```python
from build123d import *
from OCP.BRepFilletAPI import BRepFilletAPI_MakeChamfer

# Parameters (mm, degrees)
SKETCH1_W           = 60.96
SKETCH1_H           = 16.51
SKETCH1_W_2         = 50.8
SKETCH1_H_2         = 6.35
BOSS_EXTRUDE1_DEPTH = 19.05
BOSS_EXTRUDE2_DEPTH = 60.96
SKETCH7_W           = 50.8
SKETCH7_H           = 6.35
CUT_EXTRUDE1_DEPTH  = 19.05
SKETCH8_R           = 1.524
CUT_EXTRUDE2_DEPTH  = 61.718810561
SKETCH9_R           = 1.593897105
CUT_EXTRUDE3_DEPTH  = 69.202157429
CHAMFER1_SIZE       = 2.1082
CHAMFER1_SIZE2      = 1.832630301
SKETCH10_W          = 52.07
SKETCH10_H          = 7.62
CUT_EXTRUDE4_DEPTH  = 19.05
SKETCH11_W          = 52.07
SKETCH11_H          = 7.62
CUT_EXTRUDE5_DEPTH  = 19.05
CHAMFER2_SIZE       = 1.27


with BuildPart() as part:
    # Sketch1 → Boss-Extrude1 (new body)
    with BuildSketch(Plane(origin=(0, 0, 0), x_dir=(1, 0, 0), z_dir=(0, 1, 0))):
        Rectangle(SKETCH1_W, SKETCH1_H)
        Rectangle(SKETCH1_W_2, SKETCH1_H_2, mode=Mode.SUBTRACT)
    extrude(amount=BOSS_EXTRUDE1_DEPTH)

    # Sketch5 → Boss-Extrude2 (add)
    with BuildSketch(Plane(origin=(30.48, 0, 0), x_dir=(0, 0, -1), z_dir=(1, 0, 0))):
        with BuildLine():
            Line((8.255, 19.05), (-8.255, 19.05))
            Line((-8.255, 19.05), (-39.884181664, 16.282805168))
            Line((-39.884181664, 16.282805168), (-41.323122977, 32.729979633))
            Line((-41.323122977, 32.729979633), (-28.671450311, 33.836857566))
            Line((-28.671450311, 33.836857566), (-9.693941313, 35.497174465))
            ThreePointArc((-9.693941313, 35.497174465), (2.898994328, 31.222448831), (8.255, 19.05))
        make_face()
    extrude(amount=-BOSS_EXTRUDE2_DEPTH)

    # Sketch7 → Cut-Extrude1 (cut)
    with BuildSketch(Plane(origin=(0, -3.339221533, 38.167476773), x_dir=(1, 0, 0), z_dir=(0, -0.08715574274765728, 0.9961946980917457))):
        with Locations((0, 28.449053402)):
            Rectangle(SKETCH7_W, SKETCH7_H)
    extrude(amount=-CUT_EXTRUDE1_DEPTH, mode=Mode.SUBTRACT)

    # Sketch8 → Cut-Extrude2 (cut, through all)
    with BuildSketch(Plane(origin=(0, 36.069201166, 3.155646204), x_dir=(1, 0, 0), z_dir=(0, 0.9961946980917459, 0.08715574274765486))):
        with Locations(Location((0, -28.153270333, 0), (0, 0, 270))):
            Circle(SKETCH8_R)
    extrude(amount=-CUT_EXTRUDE2_DEPTH, mode=Mode.SUBTRACT)

    # Sketch9 → Cut-Extrude3 (cut, through all)
    with BuildSketch(Plane(origin=(0, 0, -8.255), x_dir=(-1, 0, 0), z_dir=(0, 0, -1))):
        with Locations((0, 10.16)):
            Circle(SKETCH9_R)
    extrude(amount=-CUT_EXTRUDE3_DEPTH, mode=Mode.SUBTRACT)

    # Chamfer1: one chamfer whose edges measure the first distance from different faces: ONE call of the kernel's chamfer builder (chamfer() names one face for all edges)
    chamfer1_edges_1 = [part.edges().sort_by_distance(p)[0] for p in [
        (0, 33.748307332, 29.683584125),
    ]]
    chamfer1_side_1 = [part.faces().sort_by_distance(p)[0] for p in [
        (0, 34.115461929, 25.486987868),
    ]]
    chamfer1_edges_2 = [part.edges().sort_by_distance(p)[0] for p in [
        (1.593897105, 10.16, -8.255),
    ]]
    chamfer1_side_2 = [part.faces().sort_by_distance(p)[0] for p in [
        (-29.841327619, 9.525, -8.255),
    ]]
    chamfer1 = BRepFilletAPI_MakeChamfer(part.part.solid().wrapped)
    for e in chamfer1_edges_1:
        chamfer1.Add(CHAMFER1_SIZE, CHAMFER1_SIZE2, e.wrapped, chamfer1_side_1[0].wrapped)  # the first distance lies on this face
    for e in chamfer1_edges_2:
        chamfer1.Add(CHAMFER1_SIZE, CHAMFER1_SIZE2, e.wrapped, chamfer1_side_2[0].wrapped)  # the first distance lies on this face
    add(Compound.cast(chamfer1.Shape()), mode=Mode.REPLACE)

    # Sketch10 → Cut-Extrude4 (cut)
    with BuildSketch(Plane(origin=(0, -3.339221533, 38.167476773), x_dir=(1, 0, 0), z_dir=(0, -0.08715574274765728, 0.9961946980917457))):
        with Locations((0, 28.449053402)):
            Rectangle(SKETCH10_W, SKETCH10_H)
    extrude(amount=-CUT_EXTRUDE4_DEPTH, mode=Mode.SUBTRACT)

    # Sketch11 → Cut-Extrude5 (cut)
    with BuildSketch(Plane.XZ):
        Rectangle(SKETCH11_W, SKETCH11_H)
    extrude(amount=-CUT_EXTRUDE5_DEPTH, mode=Mode.SUBTRACT)

    # Chamfer2
    chamfer2_edges = [part.edges().sort_by_distance(p)[0] for p in [
        (30.48, 31.222448831, -2.898994328),
        (30.48, 34.113577049, 25.508532145),
        (-30.48, 31.222448831, -2.898994328),
        (-30.48, 34.113577049, 25.508532145),
        (-30.48, 9.525, -8.255),
        (30.48, 9.525, -8.255),
    ]]
    chamfer(chamfer2_edges, length=CHAMFER2_SIZE)


solid = part.part
```
Build history of the part. All positions in model axes, mm. A direction names the side the tool comes from. Give positions to 0.01 mm unless a question says otherwise; leave off trailing zeros. Order: outer loops, then holes, each group sorted by start corner. A loop starts at its lowest first (then second) coordinate and runs counter-clockwise, first axis right, second up. Notation, with made-up numbers: M 36,16.5 L 69,16.5 A21 cw 69,29.5 Z; hole C -6.75,43 d3. An arc over 180 degrees is marked long. Return JSON: item names as keys, results as strings.
Q1. Two-plate mould, pull along Z, no slides. Class faces 1 (the face through (-30.48, 21, 12)), 2 (the face through (-0.36, 21.84, 33.07)), 3 (the face through (0.427, 17.686, 23.848)): pulls with the +Z half, pulls with the -Z half, needs draft (parallel to the pull), parting line crosses it, or undercut.
Answer list:
{"face 1": "needs draft", "face 2": "pulls with the +Z half", "face 3": "undercut"}
Q2. Flat gauge pins, fed straight in: pin 1 (3 mm diameter, centred on x = -20, z = 3, fed in from +Y); pin 2 (21 mm diameter, centred on x = -7, y = 10.5, fed in from +Z); pin 3 (1.5 mm diameter, centred on x = -11.5, z = 25.5, fed in from -Y); pin 4 (3 mm diameter, centred on x = 0, y = 10.16, fed in from -Z) (1 decimal). Where does each tip first touch, or does it go through?
Answer list:
{"pin 1": "stops at y = 35.13", "pin 2": "stops at z = 40.3", "pin 3": "stops at y = 17.48", "pin 4": "passes through"}
Q3. Band-saw the part on D-D (z = 37). Give the cut face in (x, y) (3 decimals).
Answer list:
{"outline": "M -30.48,16.535 L 30.48,16.535 L 30.48,31.833 L 29.21,33.108 L -29.21,33.108 L -30.48,31.833 Z; hole M -26.035,21.496 L 26.035,21.496 L 26.035,29.145 L -26.035,29.145 Z"}
Q4. 3-axis set-ups, long thin cutter, end or side, ignore diameter. For faces 4 (the face through (26.035, 9, 0)), 5 (the face through (30.48, 21, 12)), 6 (the face through (-0.364, 26.715, 21.674)): which of +Z, -Z, +X, -X, +Y, -Y reach the whole face in a straight line?
Answer list:
{"face 4": "-Y", "face 5": "+Z, -Z, +X, +Y, -Y", "face 6": "none"}
Q5. Band-saw the part on A-A (y = 3). Give the cut face in (x, z) (3 decimals), then the cut area to 3 significant figures.
Answer list:
{"outline": "M -30.48,-6.985 L -29.21,-8.255 L 29.21,-8.255 L 30.48,-6.985 L 30.48,8.255 L -30.48,8.255 Z; hole M -26.035,-3.81 L 26.035,-3.81 L 26.035,3.81 L -26.035,3.81 Z", "area": "608 mm^2"}
Q6. Band-saw the part on B-B (y = 10.16). Give the cut face in (x, z) (3 decimals), then the cut area to 3 significant figures.
Answer list:
{"outline": "M -30.48,-6.985 L -29.21,-8.255 L -3.702,-8.255 L -1.594,-6.422 L -1.594,-3.81 L -26.035,-3.81 L -26.035,3.81 L -1.594,3.81 L -1.594,8.255 L -30.48,8.255 Z; M 1.594,-6.422 L 3.702,-8.255 L 29.21,-8.255 L 30.48,-6.985 L 30.48,8.255 L 1.594,8.255 L 1.594,3.81 L 26.035,3.81 L 26.035,-3.81 L 1.594,-3.81 Z", "area": "576 mm^2"}
Q7. Band-saw the part on C-C (x = -21.5). Give the cut face in (y, z) (3 decimals), then the cut area to 3 significant figures.
Answer list:
{"outline": "M 0,-8.255 L 19.05,-8.255 A16.51 ccw 35.497,9.694 L 32.73,41.323 L 28.797,40.979 L 30.457,22.002 L 22.866,21.337 L 21.206,40.315 L 16.283,39.884 L 19.05,8.255 L 0,8.255 L 0,3.81 L 19.05,3.81 L 19.05,-3.81 L 0,-3.81 Z", "area": "774 mm^2"}
Q8. Wall check: probe 1 along Z at (x, y) = (26, 5.5) (3 decimals); probe 2 along Y at (x, z) = (0, -5.45); probe 3 along Y at (x, z) = (15.5, 33.5). Give the ranges that are in metal, low to high. Write a range as from..to.
Answer list:
{"probe 1": "z = -8.255..-3.81, 3.81..8.255", "probe 2": "y = 0..8.57, 11.75..28.26", "probe 3": "y = 16.84..21.8, 29.45..33.41"}
